```python
from build123d import *

# Parameters (mm, degrees)
SKETCH1_R           = 4
BOSS_EXTRUDE1_DEPTH = 5
BOSS_EXTRUDE2_DEPTH = 15
SKETCH3_R           = 7.5
SKETCH3_R_2         = 4
BOSS_EXTRUDE3_DEPTH = 5
SKETCH5_R           = 4
CUT_EXTRUDE1_DEPTH  = 5
BOSS_EXTRUDE4_START = -5
SKETCH6_R           = 7.5
BOSS_EXTRUDE4_DEPTH = 5
CUT_EXTRUDE2_START  = -5
SKETCH7_R           = 4
CUT_EXTRUDE2_DEPTH  = 5
BOSS_EXTRUDE5_DEPTH = 15
SKETCH9_R           = 7.5
BOSS_EXTRUDE6_DEPTH = 5
SKETCH10_R          = 7.5
BOSS_EXTRUDE7_DEPTH = 5
SKETCH11_R          = 4
CUT_EXTRUDE3_DEPTH  = 64
SCALE1_SCALE        = 0.7


with BuildPart() as part:
    # Sketch1 → Boss-Extrude1 (new body)
    with BuildSketch(Plane(origin=(0, 0, 0), x_dir=(0, 0, -1), z_dir=(1, 0, 0))):
        with BuildLine():
            Line((15, 0), (0, 0))
            Line((0, 0), (0, -15.59))
            ThreePointArc((0, -15.59), (1.276909506, -19.776065539), (4.672838586, -22.536737244))
            Line((4.672838586, -22.536737244), (37.484806943, -35.890449582))
            Line((37.484806943, -35.890449582), (43.13912977, -21.996975093))
            Line((43.13912977, -21.996975093), (19.672838586, -12.446737244))
            ThreePointArc((19.672838586, -12.446737244), (16.276909506, -9.686065539), (15, -5.5))
            Line((15, -5.5), (15, 0))
        make_face()
        with Locations((7.5, -16.462434129)):
            Circle(SKETCH1_R, mode=Mode.SUBTRACT)
    extrude(amount=BOSS_EXTRUDE1_DEPTH)

    # Sketch2 → Boss-Extrude2 (add)
    with BuildSketch(Plane.XY):
        with BuildLine():
            Line((0, 0), (5, 0))
            ThreePointArc((5, 0), (5.732233047, 1.767766953), (7.5, 2.5))
            ThreePointArc((7.5, 2.5), (9.267766953, 3.232233047), (10, 5))
            Line((10, 5), (10, 19.86))
            Line((10, 19.86), (5, 19.86))
            Line((5, 19.86), (5, 7.5))
            Line((5, 7.5), (0, 7.5))
            Line((0, 7.5), (0, 19.86))
            Line((0, 19.86), (-5, 19.86))
            Line((-5, 19.86), (-5, 5))
            ThreePointArc((-5, 5), (-4.267766953, 3.232233047), (-2.5, 2.5))
            ThreePointArc((-2.5, 2.5), (-0.732233047, 1.767766953), (0, 0))
        make_face()
    extrude(amount=-BOSS_EXTRUDE2_DEPTH)

    # Sketch3 → Boss-Extrude3 (add)
    with BuildSketch(Plane(origin=(10, 0, 0), x_dir=(0, 0, -1), z_dir=(1, 0, 0))):
        with Locations((7.5, 19.86)):
            Circle(SKETCH3_R)
        with Locations((7.5, 19.86)):
            Circle(SKETCH3_R_2, mode=Mode.SUBTRACT)
    extrude(amount=-BOSS_EXTRUDE3_DEPTH)

    # Sketch5 → Cut-Extrude1 (cut)
    with BuildSketch(Plane(origin=(10, 0, 0), x_dir=(0, 0, -1), z_dir=(1, 0, 0))):
        with Locations(Location((7.5, 19.86, 0), (0, 0, 90))):
            Circle(SKETCH5_R)
    extrude(amount=-CUT_EXTRUDE1_DEPTH, mode=Mode.SUBTRACT)

    # Sketch6 → Boss-Extrude4 (add)
    with BuildSketch(Plane.ZY.offset(5).offset(BOSS_EXTRUDE4_START)):
        with Locations((-7.5, 19.86)):
            Circle(SKETCH6_R)
    extrude(amount=BOSS_EXTRUDE4_DEPTH)

    # Sketch7 → Cut-Extrude2 (cut)
    with BuildSketch(Plane.ZY.offset(5).offset(CUT_EXTRUDE2_START)):
        with Locations(Location((-7.5, 19.86, 0), (0, 0, 90))):
            Circle(SKETCH7_R)
    extrude(amount=CUT_EXTRUDE2_DEPTH, mode=Mode.SUBTRACT)

    # Sketch8 → Boss-Extrude5 (add)
    with BuildSketch(Plane(origin=(0, -3.809395954, 1.55033606), x_dir=(1, 0, 0), z_dir=(0, 0.926231632569695, -0.376954855158118))):
        with BuildLine():
            Line((0, 48.248693155), (5, 48.248693155))
            Line((5, 48.248693155), (24.55634321, 57.895622609))
            ThreePointArc((24.55634321, 57.895622609), (25.552769913, 58.816883816), (25.92108759, 60.122996551))
            Line((25.92108759, 60.122996551), (25.92108759, 74.712996551))
            Line((25.92108759, 74.712996551), (20.92108759, 74.712996551))
            Line((20.92108759, 74.712996551), (20.92108759, 64.128787942))
            ThreePointArc((20.92108759, 64.128787942), (20.552769913, 62.822675208), (19.55634321, 61.901414001))
            Line((19.55634321, 61.901414001), (2.258260879, 53.528693155))
            Line((2.258260879, 53.528693155), (-14.685235236, 61.886733815))
            ThreePointArc((-14.685235236, 61.886733815), (-15.702336235, 62.808740922), (-16.079254544, 64.128787942))
            Line((-16.079254544, 64.128787942), (-16.079254544, 74.791257758))
            Line((-16.079254544, 74.791257758), (-21.079254544, 74.791257758))
            Line((-21.079254544, 74.791257758), (-21.079254544, 60.201257758))
            ThreePointArc((-21.079254544, 60.201257758), (-20.702336235, 58.881210738), (-19.685235236, 57.95920363))
            Line((-19.685235236, 57.95920363), (0, 48.248693155))
        make_face()
    extrude(amount=-BOSS_EXTRUDE5_DEPTH)

    # Sketch9 → Boss-Extrude6 (add)
    with BuildSketch(Plane(origin=(25.92108759, 0, 0), x_dir=(0, 0, -1), z_dir=(1, 0, 0))):
        with Locations((64.824043295, -38.919559991)):
            Circle(SKETCH9_R)
    extrude(amount=-BOSS_EXTRUDE6_DEPTH)

    # Sketch10 → Boss-Extrude7 (add)
    with BuildSketch(Plane.ZY.offset(21.079254544)):
        with Locations((-64.896531301, -38.949060933)):
            Circle(SKETCH10_R)
    extrude(amount=-BOSS_EXTRUDE7_DEPTH)

    # Sketch11 → Cut-Extrude3 (cut)
    with BuildSketch(Plane(origin=(25.92108759, 0, 0), x_dir=(0, 0, -1), z_dir=(1, 0, 0))):
        with Locations((64.896531301, -38.949060933)):
            Circle(SKETCH11_R)
    extrude(amount=-CUT_EXTRUDE3_DEPTH, mode=Mode.SUBTRACT)


with BuildPart() as part_1:
    # Scale1: scaled about (2.485117757, -17.850767572, -31.920196675)
    add(part.part.scale(SCALE1_SCALE).moved(Location((0.745535327, -5.355230272, -9.576059003))))


solid = part_1.part
```
Check sheet for the modelled part. Datum: model origin and axes. Units: mm. A direction names the side the tool comes from. Give positions to 0.01 mm unless a question says otherwise; leave off trailing zeros. Write each loop counter-clockwise with the first axis right and the second up, starting at its lowest first coordinate (ties: lowest second). Pieces come first, ordered by that corner, then holes. Notation, with made-up numbers: (34, 2.25) - (91, 2.25) arc R17 ccw to (91, 22.25) - close; hole circle Ø5 at (35.25, 78). An arc over 180 degrees is marked (long way). Answer as a JSON object with one key per item and string values. Group by question number.
1) Release check for a two-part mould opening along Y. For faces 4 (the face through (-0.98, 11.217, -15.667)), 5 (the face through (2.471, -12.171, -20.994)), 6 (the face through (-10.51, -30, -53)) record: pulls with the +Y half, pulls with the -Y half, needs draft (parallel to the pull), parting line crosses it, or undercut.
2) Sectioned sample at C-C (x = -4.5). Record the cut outline in (y, z).
3) Sectioned sample at A-A (y = 10). Record the cut outline in (x, z), then the cut area to 3 significant figures.
4) Access from +Z, -Z, +X, -X, +Y, -Y to the whole of each face (thin tool, end or side, straight path). Record for faces 1 (the face through (4.246, 5, -15)), 2 (the face through (-10.24, -29.39, -47.25)), 3 (the face through (0, 0, -20.076)).
5) Depth check by flat-ended pin: P1, Ø4, axis at x = 6, z = -34.5, coming from the -Y side; P2, Ø10, axis at x = 14, y = -30.5, coming from the -Z side; P3, Ø8.5, axis at y = 6.5, z = -16.5, coming from the +X side; P4, Ø4.5, axis at y = -32.62, z = -55, coming from the +X side. Enter the tip coordinate at first touch or a pass-through.
6) Sectioned sample at D-D (y = -11.5). Record the cut outline in (x, z).
7) Thickness scan on probe 1 along X at (y, z) = (-20.5, -37); probe 2 along Z at (x, y) = (-1.5, 1); probe 3 along X at (y, z) = (-33, -43.5). Record the ranges inside material, lowest first. Write a range as from..to.
8) Sectioned sample at B-B (z = -56). Record the cut outline in (x, y).
Geometry results:
{
 "1": {"face 4": "undercut", "face 5": "pulls with the +Y half", "face 6": "needs draft"},
 "2": {"outline": "(-33.14, -42.36) - (-23.42, -46.32) - (-21.73, -42.17) - (-31.45, -38.21) - close"},
 "3": {"outline": "(-2.75, -19.87) - (0.75, -19.87) - (0.75, -17.22) - (-2.75, -17.22) - close; (-2.75, -12.43) - (0.75, -12.43) - (0.75, -9.78) - (-2.75, -9.78) - close; (4.25, -19.87) - (7.75, -19.87) - (7.75, -17.22) - (4.25, -17.22) - close; (4.25, -12.43) - (7.75, -12.43) - (7.75, -9.78) - (4.25, -9.78) - close", "area": "37.1 mm^2"},
 "4": {"face 1": "+Z, -Z, +Y", "face 2": "-Z, -Y", "face 3": "-Z, +X, -X, +Y"},
 "5": {"P1": "stops at y = -30.75", "P2": "stops at z = -60.2", "P3": "stops at x = 7.75", "P4": "passes through"},
 "6": {"outline": "(0.75, -20.6) - (4.25, -20.6) - (4.25, -9.58) - (0.75, -9.58) - close"},
 "7": {"probe 1": "x = 0.75..4.25", "probe 2": "z = -20.08..-9.58", "probe 3": "x = -13.98..-6.54, 11.36..18.87"},
 "8": {"outline": "(-14.01, -37.77) - (-10.51, -37.77) - (-10.51, -35.24) - (-14.01, -35.24) - close; (-14.01, -30) - (-10.51, -30) - (-10.51, -27.36) - (-14.01, -27.36) - close; (15.39, -37.74) - (18.89, -37.74) - (18.89, -35.24) - (15.39, -35.24) - close; (15.39, -30) - (18.89, -30) - (18.89, -27.36) - (15.39, -27.36) - close"}
}
